Work out the finished part from the listing and answer in its coordinate system (mm). A direction names the side the tool comes from. Give positions to 0.01 mm unless a question says otherwise; leave off trailing zeros.
Autodesk Inventor part; units mm, degrees
ref_plane "Work Plane1" through (0, 44.45, 0) normal (0, 1, 0) x (-1, 0, 0)
ref_plane "YZ Plane" through (0, 0, 0) normal (1, 0, 0) x (0, 1, 0)
ref_plane "XY Plane" through (0, 0, 0) normal (0, 0, 1) x (1, 0, 0)
sketch "Sketch2" plane through (0, 0, 0) normal (0, 1, 0) x (-1, 0, 0)
  circle A0 centre (0, 0) radius 3.175
  line L0 (0, 0) -> (35.56, 0)
  line L1 (0, 3.175) -> (12.2611, 3.175)
  line L2 (0, -3.175) -> (12.3047, -3.175)
  line L3 (13.1799, -3.1144) -> (35.56, 0)
  line L4 (35.56, 0) -> (13.1347, 3.1146)
  arc A1 (13.1347, 3.1146) -> (12.2611, 3.175) centre (12.2611, -3.175) ccw
  arc A2 (12.3047, -3.175) -> (13.1799, -3.1144) centre (12.3047, 3.175) ccw
  circle A3 centre (0, 0) radius 1.5875
  point P0 (12.7, 3.175)
  dimension "d5" = 6.35
  dimension "d6" = 35.56
  dimension "d7" = 12.7
  dimension "d8" = 6.35
  dimension "d9" = 6.35
  dimension "d12" = 3.175
ref_plane "Work Plane1" through (0, 44.45, 0) normal (0, 1, 0) x (-1, 0, 0)
sketch "Sketch3" plane through (0, 44.45, 0) normal (0, 1, 0) x (-1, 0, 0)
  circle A0 centre (0, 0) radius 1.5875
  line L0 (0, 1.5875) -> (12.4798, 1.5875)
  line L1 (0, -1.5875) -> (12.5018, -1.5875)
  line L2 (12.9421, -1.5722) -> (35.56, 0)
  line L3 (35.56, 0) -> (12.9197, 1.5722)
  arc A1 (12.9197, 1.5722) -> (12.4798, 1.5875) centre (12.4798, -4.7625) ccw
  arc A2 (12.5018, -1.5875) -> (12.9421, -1.5722) centre (12.5018, 4.7625) ccw
  point P0 (12.7, 1.5875)
  dimension "d14" = 3.175
  dimension "d15" = 12.7
  dimension "d16" = 6.35
  dimension "d17" = 6.35
loft "Loft1" add profiles "Sketch2", "Sketch3" contours A0 | L0 L3 A2 L2 A0 | A0 L1 A1 L4 L0 | A3 / all
sketch "Sketch4" plane through (0, 0, 0) normal (0, 0, 1) x (1, 0, 0)
  line L0 (-12.2611, 0) -> (0, 0)
  line L1 (0, 0) -> (0, 12.7)
  line L2 (0, 0) -> (0, 44.45)
  line L3 (0, 12.7) -> (-7.9375, 12.7)
  line L4 (-7.9375, 12.7) -> (-7.9375, 20.6375)
  arc A0 (0, 12.7) -> (-7.9375, 20.6375) centre (-7.9375, 12.7) ccw
  line L5 (-7.9375, 20.6375) -> (-14.2875, 20.6375)
  dimension "d22" = 12.7
  dimension "d23" = 7.9375
  dimension "d24" = 7.9375
  dimension "d25" = 6.35
sketch "Sketch5" plane through (-12.3047, 0, -3.175) normal (0, -1, 0) x (1, 0, 0)
  circle A0 centre (12.3047, 3.175) radius 1.7145
  dimension "d26" = 3.429
sweep "Sweep1" cut profiles "Sketch5" path "Sketch4" path curves L1 A0 L5
sketch "Sketch6" plane through (0, 0, 0) normal (0, 0, 1) x (1, 0, 0)
  line L0 (3.175, 0) -> (0, 0)
  line L1 (3.175, 0) -> (-3.175, 0)
  line L2 (0, 0) -> (-12.3047, 0)
  line L3 (-3.175, 0) -> (3.1148, 1.6853)
  line L4 (3.175, 0) -> (1.5875, 44.45)
  dimension "d29" = 6.35
  dimension "d30" = 15
extrude "Extrusion3" cut sketch "Sketch6" along normal mid plane 25.4
properties part number "RudderUpperControlSurface"
1. Which of the six approach directions +Z, -Z, +X, -X, +Y, -Y give full straight-line access (tool end or side, diameter ignored) to faces 4 (the face through (-11.157, 19.374, -1.159)), 5 (the face through (-13, 44.45, 0))?
Findings below:
face 4: none
face 5: +Z, -Z, +X, -X, +Y
2. Straight lines are drawn through the part: probe 1 along Y at (x, z) = (-11.25, 0); probe 2 along Y at (x, z) = (-4, -1); probe 3 along Z at (x, y) = (0, 5.5). For each, find the intervals that lie inside material, in ascending order.
Findings below:
probe 1: y = 0 to 18.92, 22.35 to 44.45
probe 2: y = 0 to 17.93, 21.16 to 44.45
probe 3: z = -2.98 to -1.71, 1.71 to 2.98
3. Given P1, Ø1.5, axis at x = -13, z = 2, coming from the -Y side; P2, Ø2, axis at y = 6, z = 1.5, coming from the +X side; P3, Ø1, axis at y = 20.5, z = 0, coming from the +X side, each flat-ended and moving along its own axis, determine where each tip first touches the part or whether it passes through.
Findings below:
P1: stops at y = 0
P2: stops at x = 2.92
P3: stops at x = 2.46
4. The mould has two halves that part along Z. Classify faces 1 (the face through (2.376, 22.345, -0.052)), 2 (the face through (-1.713, 6.629, -0.075)), 3 (the face through (-16, 0, 0)): pulls with the +Z half, pulls with the -Z half, needs draft (parallel to the pull), parting line crosses it, or undercut.
Findings below:
face 1: parting line crosses it
face 2: undercut
face 3: needs draft
